Check sheet for the modelled part. Datum: model origin and axes. Units: mm. A direction names the side the tool comes from. Give positions to 0.01 mm unless a question says otherwise; leave off trailing zeros. Loops run counter-clockwise (first coordinate to the right, second up) from the corner with the lowest first, then second, coordinate; pieces in that order, holes last. Notation, with made-up numbers: M 58.5,-28.5 L 95.5,-28.5 A25 ccw 95.5,9.5 Z; hole C -2,-19.75 d5. An arc over 180 degrees is marked long. Use one line per item in the form item = value.
Autodesk Inventor part; units mm, degrees
ref_plane "Plan de départ" through (0, 0, 0) normal (0, 0, 1) x (1, 0, 0)
ref_plane "Plan de fin" through (0, 0, 370) normal (0, 0, 1) x (1, 0, 0)
ref_plane "YZ Plane" through (0, 0, 0) normal (1, 0, 0) x (0, 1, 0)
ref_plane "Plan de départ" through (0, 0, 0) normal (0, 0, 1) x (1, 0, 0)
ref_plane "Plan de fin" through (0, 0, 370) normal (0, 0, 1) x (1, 0, 0)
sketch "Esquisse" plane through (0, 0, 0) normal (0, 0, 1) x (1, 0, 0)
  line L0 (-15, -11) -> (-15, 11)
  line L1 (-11, 15) -> (11, 15)
  line L2 (15, 11) -> (15, -11)
  line L3 (11, -15) -> (-11, -15)
  arc A0 (-15, -11) -> (-11, -15) centre (-11, -11) ccw
  arc A1 (15, 11) -> (11, 15) centre (11, 11) ccw
  arc A2 (-11, 15) -> (-15, 11) centre (-11, 11) ccw
  arc A3 (11, -15) -> (15, -11) centre (11, -11) ccw
  arc A4 (-11, 13) -> (-13, 11) centre (-11, 11) ccw
  line L4 (-11, 13) -> (11, 13)
  arc A5 (13, 11) -> (11, 13) centre (11, 11) ccw
  line L5 (13, 11) -> (13, -11)
  arc A6 (11, -13) -> (13, -11) centre (11, -11) ccw
  line L6 (11, -13) -> (-11, -13)
  arc A7 (-13, -11) -> (-11, -13) centre (-11, -11) ccw
  line L7 (-13, -11) -> (-13, 11)
  line L8 (0, 22.1598) -> (0, -22.1598) construction
  line L9 (-22.1598, 0) -> (22.1598, 0) construction
  dimension "d7" = 4
  dimension "d9" = 30
  dimension "d11" = 30
  dimension "d12" = 2
  dimension "d15" = 15
  dimension "d16" = 15
extrude "Corps" add sketch "Esquisse" along normal up to surface (370 mm away) from surface at 0
sketch "Sketch3" plane through (0, 0, 0) normal (0, 0, 1) x (1, 0, 0)
  line L0 (0, 0) -> (10, 0)
ref_plane "Work Plane3" through (0, 0, 0) normal (0, -1, 0) x (1, 0, 0)
sketch "Sketch4" plane through (0, 0, 0) normal (0, -1, 0) x (1, 0, 0)
  line L0 (-2, 0) -> (12, 0)
  line L1 (-2, 370) -> (12, 370)
  dimension "d18" = 370
equation "\"d7\" = G_IR"
equation "\"d9\" = G_W"
equation "\"d11\" = G_H"
equation "\"d12\" = G_T"
equation "\"d15\" = 0.5 * d9"
equation "\"d16\" = 0.5 * d11"
equation "\"d3\" = G_L"
equation "\"G_W\" = 30"
equation "\"G_H\" = 30"
equation "\"G_T\" = 2"
equation "\"G_IR\" = 4"
equation "\"G_L\" = d18"
equation "\"G_OFFSET_START\" = 0"
equation "\"G_OFFSET_END\" = 0"
properties part number "ISO 10799-2 - 30x30x2 - 370" material "Acier, doux"
1) Release check for a two-part mould opening along Y. For faces 1 (the face through (13, 0, 182)), 2 (the face through (-14, 0, 370)), 3 (the face through (0, -15, 182)), 4 (the face through (0, 15, 182)) record: pulls with the +Y half, pulls with the -Y half, needs draft (parallel to the pull), parting line crosses it, or undercut.
Evaluation:
face_1 = undercut
face_2 = needs draft
face_3 = pulls with the -Y half
face_4 = pulls with the +Y half
2) Section check A-A (y = 3.75). Record the cut outline in (x, z).
Evaluation:
outline = M -15,0 L -13,0 L -13,370 L -15,370 Z; M 13,0 L 15,0 L 15,370 L 13,370 Z
3) Set-up check for faces 5 (the face through (0, -13, 182)), 6 (the face through (-15, 0, 182)): record each of +Z, -Z, +X, -X, +Y, -Y from which the full face is reachable in a straight line by a thin tool's end or side.
Evaluation:
face_5 = +Z, -Z
face_6 = +Z, -Z, -X, +Y, -Y
4) Section check B-B (z = 336). Record the cut outline in (x, y), then the cut area to 3 significant figures.
Evaluation:
outline = M -15,-11 A4 ccw -11,-15 L 11,-15 A4 ccw 15,-11 L 15,11 A4 ccw 11,15 L -11,15 A4 ccw -15,11 Z; hole M -13,-11 A2 ccw -11,-13 L 11,-13 A2 ccw 13,-11 L 13,11 A2 ccw 11,13 L -11,13 A2 ccw -13,11 Z
area = 214 mm^2
5) Scan lines: line 1 (Y direction, x = -7.25, z = 202.5); line 2 (X direction, y = -11.5, z = 148). Record each from-to range of solid material in increasing order.
Evaluation:
line_1 = -15 to -13, 13 to 15
line_2 = -14.97 to -12.94, 12.94 to 14.97
